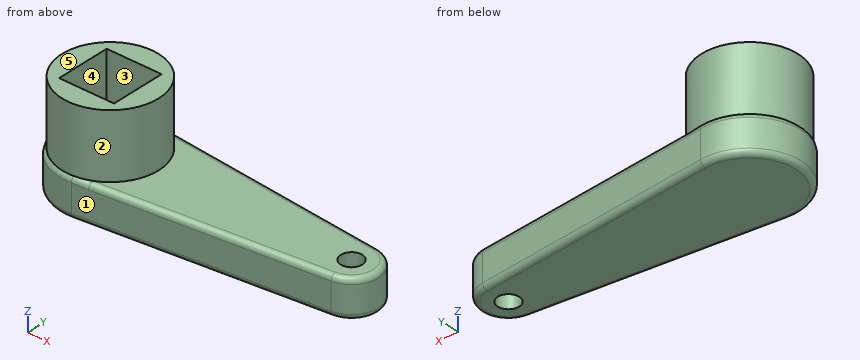
from build123d import *

# Parameters (mm, degrees)
F1_DEPTH = 7
F2_R     = 2
F3_DEPTH = 25
F2_R_2   = 9
F2_W     = 10.25
F2_H     = 10.25
F4_DEPTH = 12
F5_R     = 1


with BuildPart() as f1:
    # F0 (on Top) → F1 (new body)
    with BuildSketch(Plane.XY):
        with BuildLine():
            Line((45.5, 4.974937), (0.95, 9.452381))
            ThreePointArc((0.95, 9.452381), (-9.5, 0), (0.95, -9.452381))
            Line((0.95, -9.452381), (45.5, -4.974937))
            ThreePointArc((45.5, -4.974937), (50, 0), (45.5, 4.974937))
        make_face()
    extrude(amount=F1_DEPTH)

    # F2 (on face) → F3 (cut)
    with BuildSketch(Plane.XY.offset(7)):
        with Locations((45, 0)):
            Circle(F2_R)
    extrude(amount=-F3_DEPTH, mode=Mode.SUBTRACT)

    # F2 (on face) → F4 (join)
    with BuildSketch(Plane.XY.offset(7)):
        Circle(F2_R_2)
        Rectangle(F2_W, F2_H, mode=Mode.SUBTRACT)
    extrude(amount=F4_DEPTH)

    # F5
    f5_edges = [f1.edges().sort_by_distance(p)[0] for p in [
        (23.225, -7.213659, 0),
        (23.225, -7.213659, 7),
    ]]
    fillet(f5_edges, radius=F5_R)


solid = f1.part
Model file for the job. Use its own axes, mm. Face numbers are marked on the shaded views. A direction names the side the tool comes from. Give positions to 0.01 mm unless a question says otherwise; leave off trailing zeros. Loops run counter-clockwise (first coordinate to the right, second up) from the corner with the lowest first, then second, coordinate; pieces in that order, holes last. Notation, with made-up numbers: (-2.5, -18) -> (55.5, -18) arc R33 cw to (55.5, 20) -> close; hole circle Ø4 at (-24, -33). An arc over 180 degrees is marked (long way). Use a Markdown table: item, result. Add a question column.
(1) Wall check: line 1 along Y through (x, z) = (0, 13) (3 decimals); line 2 along Z through (x, y) = (21, 0.5); line 3 along Y through (x, z) = (45, 5). Give the ranges that are in metal, low to high.
(2) Tool access for the marked faces 4 and 5: list every direction of +Z, -Z, +X, -X, +Y, -Y with a clear straight run to the whole face (end or side of a thin tool).
(3) Slice it at A-A on z = 9. List the corners of the cut face in (x, y) (3 decimals).
(4) Slice it at B-B on z = 4. List the corners of the cut face in (x, y).
(5) Drop flat-ended pins along their axis: pin 1 Ø3 at (y, z) = (7, 16.5) entering from +X; pin 2 Ø4 at (x, z) = (42, 4) entering from -Y; pin 3 Ø2 at (x, z) = (-2.5, 11) entering from -Y; pin 4 Ø5 at (x, y) = (45, 0) entering from -Z. Give the stop position or say it passes through.
(6) Mould opens along Y. For the marked faces 1, 2 and 3 say: +Y half, -Y half, draft (parallel to the pull), parting line (faces both ways), or undercut.
Filled sheet:
| question | item | result |
|---|---|---|
| 1 | line 1 | -9 to -5.125, 5.125 to 9 |
| 1 | line 2 | 0 to 7 |
| 1 | line 3 | -5.03 to -2, 2 to 5.03 |
| 2 | face 4 | +Z |
| 2 | face 5 | +Z, +X, -X, +Y, -Y |
| 3 | outline | circle Ø18 at (0, 0); hole (-5.125, -5.125) -> (5.125, -5.125) -> (5.125, 5.125) -> (-5.125, 5.125) -> close |
| 4 | outline | (0.95, -9.45) -> (45.5, -4.97) arc R5 ccw to (45.5, 4.97) -> (0.95, 9.45) arc R9.5 ccw (long way) to start; hole circle Ø4 at (45, 0) |
| 5 | pin 1 | x = 7.12 |
| 5 | pin 2 | y = -5.53 |
| 5 | pin 3 | y = -8.87 |
| 5 | pin 4 | z = 0 |
| 6 | face 1 | -Y half |
| 6 | face 2 | parting line |
| 6 | face 3 | undercut |
